```python
from build123d import *

# Parameters (mm, degrees)
SKETCH1_R           = 9.6
SKETCH1_R_2         = 4.2
BOSS_EXTRUDE1_DEPTH = 2
SKETCH4_W           = 60
SKETCH4_H           = 58
SKETCH4_R           = 2
SKETCH4_R_2         = 9.6
BOSS_EXTRUDE3_DEPTH = 2
SKETCH5_R           = 3
CUT_EXTRUDE1_DEPTH  = 4


with BuildPart() as part:
    # Sketch1 → Boss-Extrude1 (new body)
    with BuildSketch(Plane.XY):
        with BuildLine():
            Line((40, 29), (20, 29))
            Line((20, 29), (20, 15.95))
            Line((20, 15.95), (13.75, 15.95))
            ThreePointArc((13.75, 15.95), (10.780151519, 17.180151519), (9.55, 20.15))
            Line((9.55, 20.15), (9.55, 29))
            Line((9.55, 29), (-9.55, 29))
            Line((-9.55, 29), (-9.55, 20.15))
            ThreePointArc((-9.55, 20.15), (-10.780151519, 17.180151519), (-13.75, 15.95))
            Line((-13.75, 15.95), (-20, 15.95))
            Line((-20, 15.95), (-20, -16.278610808))
            Line((-20, -16.278610808), (-16.186, -16.278610808))
            Line((-16.186, -16.278610808), (-12.112917629, -13.378610808))
            ThreePointArc((-12.112917629, -13.378610808), (-6.255528438, -14.364), (-7.240917629, -20.221389192))
            Line((-7.240917629, -20.221389192), (-11.314, -23.121389192))
            Line((-11.314, -23.121389192), (-11.314, -29))
            Line((-11.314, -29), (9.55, -29))
            Line((9.55, -29), (9.55, -19.7))
            ThreePointArc((9.55, -19.7), (10.780151519, -16.730151519), (13.75, -15.5))
            Line((13.75, -15.5), (20, -15.5))
            Line((20, -15.5), (20, -29))
            Line((20, -29), (40, -29))
            Line((40, -29), (40, 29))
        make_face()
        with Locations((0, 8.8)):
            Circle(SKETCH1_R, mode=Mode.SUBTRACT)
        with Locations((-5.725, -6.1)):
            Circle(SKETCH1_R_2, mode=Mode.SUBTRACT)
        with Locations((5.725, -6.1)):
            Circle(SKETCH1_R_2, mode=Mode.SUBTRACT)
    extrude(amount=BOSS_EXTRUDE1_DEPTH)

    # Sketch4 → Boss-Extrude3 (add)
    with BuildSketch(Plane.XY.offset(2)):
        with Locations((10, 0)):
            Rectangle(SKETCH4_W, SKETCH4_H)
        with Locations((13.75, -19.7)):
            Circle(SKETCH4_R, mode=Mode.SUBTRACT)
        with Locations((-13.75, 20.15)):
            Circle(SKETCH4_R, mode=Mode.SUBTRACT)
        with Locations((13.75, 20.15)):
            Circle(SKETCH4_R, mode=Mode.SUBTRACT)
        with Locations((-13.75, -19.7)):
            Circle(SKETCH4_R, mode=Mode.SUBTRACT)
        with Locations((0, 8.8)):
            Circle(SKETCH4_R_2, mode=Mode.SUBTRACT)
    extrude(amount=BOSS_EXTRUDE3_DEPTH)

    # Sketch5 → Cut-Extrude1 (cut)
    with BuildSketch(Plane.XY.offset(4)):
        with Locations((28, 15)):
            Circle(SKETCH5_R)
        with Locations((28, -15)):
            Circle(SKETCH5_R)
    extrude(amount=-CUT_EXTRUDE1_DEPTH, mode=Mode.SUBTRACT)


solid = part.part
```
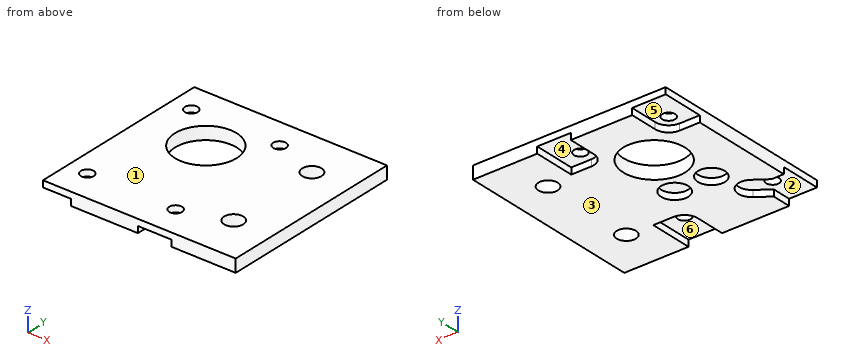
Can you work these out from the model? Positions are in its coordinate system, mm. Face numbers are marked on the shaded views. A direction names the side the tool comes from. Coordinates: 2 decimals unless noted, no trailing zeros. Loops run counter-clockwise (first coordinate to the right, second up) from the corner with the lowest first, then second, coordinate; pieces in that order, holes last.
1) Imagine slicing it at B-B on z = 1.1. List the corners of the cut face in (x, y) for me (3 decimals), plus the area to 3 significant figures.
2) Imagine slicing it at D-D on y = 8.8. List the corners of the cut face in (x, z) for me.
3) Which directions (+Z, -Z, +X, -X, +Y, -Y) give clear straight access to the entire face, cutting with the end or side of a thin tool? Please do the marked faces 3, 4, 5 and 6.
4) Imagine slicing it at A-A on x = 0. List the corners of the cut face in (y, z) for me, plus the area to 3 significant figures.
5) I need wall thicknesses on probe 1 along Y at (x, z) = (28, 1.5); probe 2 along Y at (x, z) = (-13.75, 2.75); probe 3 along X at (y, z) = (8, 3.55). Which ranges of each line are inside material? Lowest first, please.
6) Imagine slicing it at C-C on x = 28. List the corners of the cut face in (y, z) for me, plus the area to 3 significant figures.
7) Thinking about a two-plate mould opening in Y: for the marked faces 1 and 2, which applies, pulls with the +Y half, pulls with the -Y half, needs draft (parallel to the pull), parting line crosses it, or undercut?
8) For pin 1 (2.5 mm diameter, centred on x = 6.5, y = -4.5, fed in from -Z); pin 2 (1.6 mm diameter, centred on y = -26, z = 1, fed in from -X); pin 3 (0.6 mm diameter, centred on x = -17, z = 1.5, fed in from +Y); pin 4 (15.5 mm diameter, centred on x = 0, y = 8.8, fed in from +Z), each with a flat end and sliding along its axis, tell me the tip position at first contact or that it passes through.
Completed:
1. outline: (-20, -16.279) - (-16.186, -16.279) - (-12.113, -13.379) arc R4.2 cw to (-7.241, -20.221) - (-11.314, -23.121) - (-11.314, -29) - (9.55, -29) - (9.55, -19.7) arc R4.2 cw to (13.75, -15.5) - (20, -15.5) - (20, -29) - (40, -29) - (40, 29) - (20, 29) - (20, 15.95) - (13.75, 15.95) arc R4.2 cw to (9.55, 20.15) - (9.55, 29) - (-9.55, 29) - (-9.55, 20.15) arc R4.2 cw to (-13.75, 15.95) - (-20, 15.95) - close; hole circle Ø8.4 at (-5.725, -6.1); hole circle Ø19.2 at (0, 8.8); hole circle Ø8.4 at (5.725, -6.1); hole circle Ø6 at (28, -15); hole circle Ø6 at (28, 15)
1. area: 2,460 mm2
2. outline: (-20, 0) - (-9.6, 0) - (-9.6, 4) - (-20, 4) - close; (9.6, 0) - (40, 0) - (40, 4) - (9.6, 4) - close
3. face 3: -Z, +X, -X, +Y, -Y
3. face 4: -Z, +Y
3. face 5: -Z, -X, +Y
3. face 6: -Z, -Y
4. outline: (-29, 0) - (-0.8, 0) - (-0.8, 4) - (-29, 4) - close; (18.4, 0) - (29, 0) - (29, 4) - (18.4, 4) - close
4. area: 155 mm2
5. probe 1: y = -29 to -18, -12 to 12, 18 to 29
5. probe 2: y = -29 to -21.7, -17.7 to 18.15, 22.15 to 29
5. probe 3: x = -20 to -9.57, 9.57 to 40
6. outline: (-29, 0) - (-18, 0) - (-18, 4) - (-29, 4) - close; (-12, 0) - (12, 0) - (12, 4) - (-12, 4) - close; (18, 0) - (29, 0) - (29, 4) - (18, 4) - close
6. area: 184 mm2
7. face 1: needs draft
7. face 2: undercut
8. pin 1: stops at z = 2
8. pin 2: stops at x = -11.31
8. pin 3: stops at y = 15.95
8. pin 4: passes through
